Here's the drawing with two shaded views (mm, measured from the low corner). I have some questions. Round coordinates to 2 decimals unless told otherwise and drop trailing zeros. Loops run counter-clockwise (first coordinate to the right, second up) from the corner with the lowest first, then second, coordinate; pieces in that order, holes last.
(1) I want a section at D-D on y = 4. Write out the boundary of the cut face in (x, z).
(2) Will these pins go through, and if not, where does the flat tip stop? pin 1 Ø7 at (x, y) = (36, 4) entering from -Z; pin 2 Ø3.5 at (x, y) = (4, 4) entering from +Z.
(3) I want a section at C-C on z = 2. Write out the boundary of the cut face in (x, y).
(4) If I drill on line 1 along Y through (x, z) = (4, 4); line 2 along X through (y, z) = (35, 2.75); line 3 along X through (y, z) = (20.5, 9.25), over which ranges is the centre line in solid material (lowest first)?
(5) Thinking about a two-plate mould opening in X: for the marked faces 1, 2 and 3, which applies, released by +X, released by -X, zero draft, split by the parting line, or undercut?
(6) I want a section at A-A on x = 12.5. Write out the boundary of the cut face in (y, z).
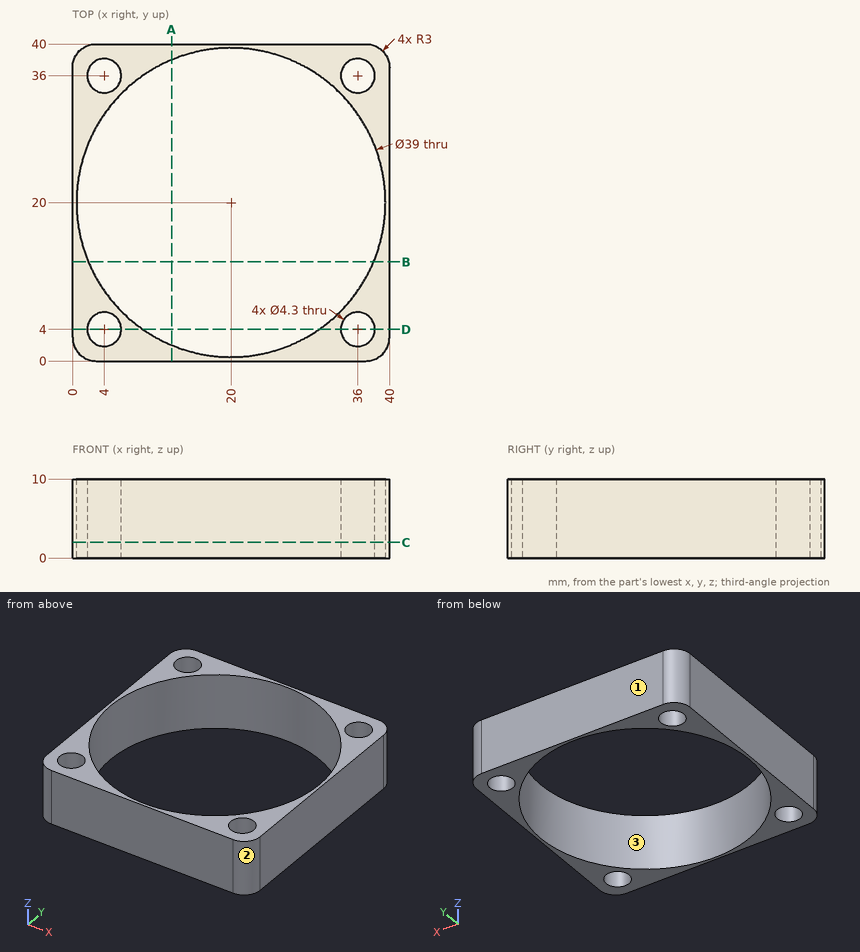
Filled sheet:
1. outline: (0, 0) - (1.85, 0) - (1.85, 10) - (0, 10) - close; (6.15, 0) - (8.85, 0) - (8.85, 10) - (6.15, 10) - close; (31.15, 0) - (33.85, 0) - (33.85, 10) - (31.15, 10) - close; (38.15, 0) - (40, 0) - (40, 10) - (38.15, 10) - close
2. pin 1: stops at z = 0
2. pin 2: passes through
3. outline: (0, 3) arc R3 ccw to (3, 0) - (37, 0) arc R3 ccw to (40, 3) - (40, 37) arc R3 ccw to (37, 40) - (3, 40) arc R3 ccw to (0, 37) - close; hole circle Ø39 at (20, 20); hole circle Ø4.3 at (4, 4); hole circle Ø4.3 at (4, 36); hole circle Ø4.3 at (36, 4); hole circle Ø4.3 at (36, 36)
4. line 1: y = 0 to 1.85, 6.15 to 8.85, 31.15 to 33.85, 38.15 to 40
4. line 2: x = 0 to 2.1, 5.9 to 7.54, 32.46 to 34.1, 37.9 to 40
4. line 3: x = 0 to 0.51, 39.49 to 40
5. face 1: zero draft
5. face 2: released by +X
5. face 3: undercut
6. outline: (0, 0) - (2, 0) - (2, 10) - (0, 10) - close; (38, 0) - (40, 0) - (40, 10) - (38, 10) - close
